Autodesk Inventor part; units mm, degrees
ref_plane "YZ Plane" through (0, 0, 0) normal (1, 0, 0) x (0, 1, 0)
ref_plane "XZ Plane" through (0, 0, 0) normal (0, 1, 0) x (-1, 0, 0)
ref_plane "XY Plane" through (0, 0, 0) normal (0, 0, 1) x (1, 0, 0)
sketch "Skizze1" plane through (0, 0, 0) normal (0, 0, 1) x (1, 0, 0)
  line L0 (-273.7, 0) -> (273.7, 0)
  line L1 (0, -189.7) -> (0, 189.7)
  line L2 (-195.5, 135.5) -> (195.5, 135.5)
  line L3 (195.5, 135.5) -> (195.5, -135.5)
  line L4 (195.5, -135.5) -> (-195.5, -135.5)
  line L5 (-195.5, -135.5) -> (-195.5, 135.5)
  point P0 (0, 0)
  dimension "d0" = 391
  dimension "d1" = 271
extrude "Extrusion1" add sketch "Skizze1" against normal blind 2
sketch "Skizze2" plane through (0, 0, 0) normal (0, 0, 1) x (1, 0, 0)
  line L0 (-190.5, 130.5) -> (190.5, 130.5)
  line L1 (190.5, 130.5) -> (190.5, -130.5)
  line L2 (190.5, -130.5) -> (-190.5, -130.5)
  line L3 (-190.5, -130.5) -> (-190.5, 130.5)
  line L4 (195.5, -135.5) -> (195.5, 135.5)
  line L5 (195.5, 135.5) -> (-195.5, 135.5)
  line L6 (-195.5, 135.5) -> (-195.5, -135.5)
  line L7 (-195.5, -135.5) -> (195.5, -135.5)
  point P0 (0, 0)
  dimension "d12" = 5
  dimension "d13" = 5
  dimension "d14" = 5
  dimension "d15" = 5
extrude "Extrusion2" add sketch "Skizze2" along normal blind 2
sketch "Skizze3" plane through (0, 0, 2) normal (0, 0, 1) x (1, 0, 0)
  line L0 (-200.5, 140.5) -> (200.5, 140.5)
  line L1 (200.5, 140.5) -> (200.5, -140.5)
  line L2 (200.5, -140.5) -> (-200.5, -140.5)
  line L3 (-200.5, -140.5) -> (-200.5, 140.5)
  line L4 (195.5, 135.5) -> (-195.5, 135.5)
  line L5 (-195.5, -135.5) -> (195.5, -135.5)
  line L6 (195.5, -135.5) -> (195.5, 135.5)
  line L7 (-195.5, 135.5) -> (-195.5, -135.5)
  point P0 (0, 0)
  dimension "d18" = 5
  dimension "d19" = 5
  dimension "d20" = 5
  dimension "d21" = 5
extrude "Extrusion3" add sketch "Skizze3" against normal blind 2
properties part number "Deckel"
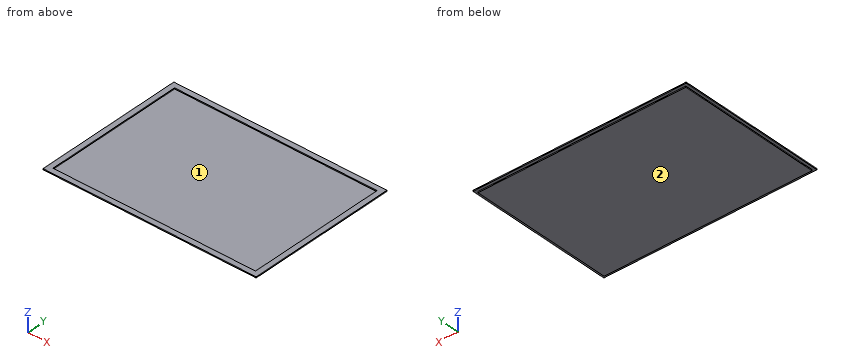
Geometry: final body of the model. Coordinates: model frame, mm. Face numbers are marked on the shaded views. Round coordinates to 2 decimals unless told otherwise and drop trailing zeros. Order: outer loops, then holes, each group sorted by start corner. A loop starts at its lowest first (then second) coordinate and runs counter-clockwise, first axis right, second up. Notation, with made-up numbers: (-19, 55) -> (40, 55) arc R31 ccw to (40, 83) -> close; hole circle Ø3 at (67.5, 25.5). An arc over 180 degrees is marked (long way). Use CSV: the item, a comma, the result in double quotes. Start each with the question number.
1) Draft query along Y for the marked faces 1 and 2. Return one class per face: +Y half, -Y half, draft (parallel to the pull), parting line (faces both ways), or undercut.
2) Section A-A (z = 0.9). Return the cut outline in (x, y).
3) Section B-B (x = 47.5). Return the cut outline in (y, z), and give its area (3 significant figures).
4) Material intervals for line 1 along X through (y, z) = (-12, 1.75); line 2 along Y through (x, z) = (134, 1.45); line 3 along Z through (x, y) = (-159, 34), sorted ascending. Write a range as from..to.
5) First-contact query: pin 1 Ø0.6 at (y, z) = (-65, -0.5) entering from -X; pin 2 Ø1.5 at (x, z) = (44.5, -1.5) entering from -Y; pin 3 Ø10 at (x, y) = (-114, -7) entering from +Z. Flat tips, straight axial feed; report the tip coordinate or a pass-through.
6) Section C-C (y = -35). Return the cut outline in (x, z).
Returned:
1,face 1,"undercut"
1,face 2,"draft"
2,outline,"(-200.5, -140.5) -> (200.5, -140.5) -> (200.5, 140.5) -> (-200.5, 140.5) -> close; hole (-190.5, -130.5) -> (190.5, -130.5) -> (190.5, 130.5) -> (-190.5, 130.5) -> close"
3,outline,"(-140.5, 0) -> (-135.5, 0) -> (-135.5, -2) -> (135.5, -2) -> (135.5, 0) -> (140.5, 0) -> (140.5, 2) -> (130.5, 2) -> (130.5, 0) -> (-130.5, 0) -> (-130.5, 2) -> (-140.5, 2) -> close"
3,area,"582 mm²"
4,line 1,"x = -200.5..-190.5, 190.5..200.5"
4,line 2,"y = -140.5..-130.5, 130.5..140.5"
4,line 3,"z = -2..0"
5,pin 1,"stops at x = -195.5"
5,pin 2,"stops at y = -135.5"
5,pin 3,"stops at z = 0"
6,outline,"(-200.5, 0) -> (-195.5, 0) -> (-195.5, -2) -> (195.5, -2) -> (195.5, 0) -> (200.5, 0) -> (200.5, 2) -> (190.5, 2) -> (190.5, 0) -> (-190.5, 0) -> (-190.5, 2) -> (-200.5, 2) -> close"
